```python
from build123d import *

# Parameters (mm, degrees)
F0_R     = 3.175
F1_DEPTH = 3.048


with BuildPart() as f1:
    # F0 (on Front) → F1 (new body)
    with BuildSketch(Plane.XZ):
        with BuildLine():
            ThreePointArc((0.6794904459, -9.5007324841), (6.9712901065, -6.4905114784), (9.525, 0))
            ThreePointArc((9.525, 0), (0, 9.525), (-9.525, 0))
            ThreePointArc((-9.525, 0), (-6.7351920908, -6.7351920908), (0, -9.525))
            Line((0, -9.525), (0.6794904459, -9.5007324841))
        make_face()
        Circle(F0_R, mode=Mode.SUBTRACT)
        with BuildLine():
            ThreePointArc((-9.525, 0), (0, 9.525), (9.525, 0))
            ThreePointArc((9.525, 0), (6.9712901065, -6.4905114784), (0.6794904459, -9.5007324841))
            Line((0.6794904459, -9.5007324841), (44.45, -7.9375))
            ThreePointArc((44.45, -7.9375), (36.5125, 0), (44.45, 7.9375))
            Line((44.45, 7.9375), (23.5403527632, 8.6871518144))
            ThreePointArc((23.5403527632, 8.6871518144), (18.1037372263, 11.1122342659), (15.875, 16.6322472884))
            Line((15.875, 16.6322472884), (15.875, 63.5))
            ThreePointArc((15.875, 63.5), (-1.0061676981, 47.6569178642), (-15.7474568899, 65.5082894468))
            Line((-15.7474568899, 65.5082894468), (-16.0035761028, 63.5))
            Line((-16.0035761028, 63.5), (-9.525, 0))
        make_face()
        with BuildLine():
            ThreePointArc((0, -9.525), (0.3399618281, -9.5189311877), (0.6794904459, -9.5007324841))
            Line((0.6794904459, -9.5007324841), (0, -9.525))
        make_face()
        with BuildLine():
            ThreePointArc((44.45, 7.9375), (36.5125, 0), (44.45, -7.9375))
            ThreePointArc((44.45, -7.9375), (50.0626600757, -5.6126600757), (52.3875, 0))
            ThreePointArc((52.3875, 0), (50.0626600757, 5.6126600757), (44.45, 7.9375))
        make_face()
        with Locations((44.45, 0)):
            Circle(F0_R, mode=Mode.SUBTRACT)
        with BuildLine():
            Line((-9.525, 114.3), (-15.7474568899, 65.5082894468))
            ThreePointArc((-15.7474568899, 65.5082894468), (-0.9666945407, 79.3455396457), (15.3865384615, 67.4076923077))
            Line((15.3865384615, 67.4076923077), (9.525, 114.3))
            ThreePointArc((9.525, 114.3), (0, 104.775), (-9.525, 114.3))
        make_face()
        with Locations((-1.5875, 100.0252)):
            Circle(F0_R, mode=Mode.SUBTRACT)
        with BuildLine():
            ThreePointArc((15.3865384615, 67.4076923077), (-0.9666945407, 79.3455396457), (-15.7474568899, 65.5082894468))
            ThreePointArc((-15.7474568899, 65.5082894468), (-1.0061676981, 47.6569178642), (15.875, 63.5))
            Line((15.875, 63.5), (15.3865384615, 67.4076923077))
        make_face()
        with Locations((0, 63.5)):
            Circle(F0_R, mode=Mode.SUBTRACT)
        with BuildLine():
            ThreePointArc((15.875, 63.5), (15.7524112928, 65.4690514116), (15.3865384615, 67.4076923077))
            Line((15.3865384615, 67.4076923077), (15.875, 63.5))
        make_face()
        with BuildLine():
            ThreePointArc((9.525, 114.3), (0, 123.825), (-9.525, 114.3))
            ThreePointArc((-9.525, 114.3), (0, 104.775), (9.525, 114.3))
        make_face()
        with Locations((0, 114.3)):
            Circle(F0_R, mode=Mode.SUBTRACT)
    extrude(amount=F1_DEPTH)


solid = f1.part
```
Work out the finished part from the listing and answer in its coordinate system (mm). A direction names the side the tool comes from. Coordinates: 2 decimals unless noted, no trailing zeros. Loops run counter-clockwise (first coordinate to the right, second up) from the corner with the lowest first, then second, coordinate; pieces in that order, holes last. Notation, with made-up numbers: M 80,49.25 L 96,49.25 A11 cw 96,60.25 Z; hole C 45.5,78.5 d4. An arc over 180 degrees is marked long. Use CSV: the item, a comma, the result in double quotes. Start each with the question number.
(1) Consider line 1 (Z direction, x = 2, y = -0.85); line 2 (X direction, y = -0.3, z = 101); line 3 (X direction, y = -1.7, z = 62) (3 decimals). Determine where each line is inside the solid, lowest interval first.
(2) For a pull along X with two mould halves and no side action, classify faces 3 (the face through (-12.81, -1.5, 32.19)), 4 (the face through (18.163, -1.503, 11.051)), 5 (the face through (41.28, -1.5, 0.14)), 6 (the face through (3, 0, 43)) as +X half, -X half, draft (parallel to the pull), parting line (faces both ways), or undercut.
(3) Find section B-B, the plane x = 33.5. Give the vertices of the cut face in (y, z), then the cut area to 3 significant figures.
(4) Given pin 1 Ø0.9 at (y, z) = (-1.5, 45) entering from +X (3 decimals); pin 2 Ø1.5 at (x, y) = (36, -2) entering from +Z, each flat-ended and moving along its own axis, determine where each tip first touches the part or whether it passes through.
(5) Find section A-A, the plane y = -1.3. State how many separate pieces and enclosed holes the cut face has, then the cut area to 3 significant figures.
(6) Find section C-C, the plane z = 71. Give the vertices of the cut face in (x, y).
(7) For faces 1 (the face through (3, -3.048, 43)), 2 (the face through (15.875, -2, 40)), determine the directions among +Z, -Z, +X, -X, +Y, -Y from which every point of the face is accessible in a straight line to the end or side of a thin tool.
Recorded:
1,line 1,"z = -9.45 to -2.47, 2.47 to 61.03, 65.97 to 111.83, 116.77 to 123.61"
1,line 2,"x = -11.22 to -4.61, 1.43 to 11.19"
1,line 3,"x = -15.851 to -2.798, 2.798 to 15.875"
2,face 3,"-X half"
2,face 4,"+X half"
2,face 5,"undercut"
2,face 6,"draft"
3,outline,"M -3.05,-8.33 L 0,-8.33 L 0,8.33 L -3.05,8.33 Z"
3,area,"50.8 mm^2"
4,pin 1,"stops at x = 15.875"
4,pin 2,"stops at z = 8.27"
5,separate pieces,"1"
5,enclosed holes,"5"
5,area,"3,910 mm^2"
6,outline,"M -15.05,-3.05 L 14.94,-3.05 L 14.94,0 L -15.05,0 Z"
7,face 1,"+Z, -Z, +X, -X, -Y"
7,face 2,"+Z, +X, +Y, -Y"
